Autodesk Inventor part; units mm, degrees
ref_plane "YZ Plane" through (0, 0, 0) normal (1, 0, 0) x (0, 1, 0)
ref_plane "XZ Plane" through (0, 0, 0) normal (0, 1, 0) x (-1, 0, 0)
ref_plane "XY Plane" through (0, 0, 0) normal (0, 0, 1) x (1, 0, 0)
sketch "Sketch1" plane through (0, 0, 0) normal (0, 0, 1) x (1, 0, 0)
  line L0 (0, 0) -> (27, 0) construction
  line L1 (27, 0) -> (27, 27)
  line L2 (27, 27) -> (0, 27)
  line L3 (0, 27) -> (0, 0) construction
  line L4 (-27, 0) -> (-27, 27)
  line L5 (-27, 27) -> (0, 27)
  line L6 (27, 0) -> (27, -27)
  line L7 (27, -27) -> (0, -27)
  line L8 (-27, -27) -> (0, -27)
  line L9 (-27, 0) -> (-27, -27)
  dimension "d0" = 27
extrude "Extrusion1" add sketch "Sketch1" along normal mid plane 138
sketch "Sketch2" plane through (0, 0, 69) normal (0, 0, 1) x (1, 0, 0)
  line L0 (27, -27) -> (27, 27)
  line L1 (27, 27) -> (-27, 27)
  line L2 (-27, 27) -> (-27, -27)
  line L3 (-27, -27) -> (27, -27)
  circle A0 centre (0, 0) radius 27
extrude "Extrusion2" cut sketch "Sketch2" against normal blind 30 contours L3 A0 L0 | A0 L1 L0 | L3 L2 A0 | A0 L2 L1
sketch "Sketch3" plane through (-27, -27, -69) normal (0, -1, 0) x (1, 0, 0)
  line L0 (54, 108) -> (54, 0)
  circle A0 centre (27, 69) radius 27
extrude "Extrusion3" add sketch "Sketch3" along normal blind 12
move or copy body "Move Body1" bodies to move or copy 1 copy no rotation origin (0, 0, 0) rotation axis (1, 0, 0) rotation angle 90
move or copy body "Move Body2" bodies to move or copy 1 copy no rotation origin (0, 0, 0) rotation axis (0, 0, 1) rotation angle 90
properties part number "Sholder_Roll"
CAD build for the part. Positions are in the model's coordinates, mm. A direction names the side the tool comes from. Give positions to 0.01 mm unless a question says otherwise; leave off trailing zeros. Order: outer loops, then holes, each group sorted by start corner. A loop starts at its lowest first (then second) coordinate and runs counter-clockwise, first axis right, second up. Notation, with made-up numbers: M 64,25.25 L 97,25.25 A36 ccw 97,63.25 Z; hole C -2,-14.5 d2. An arc over 180 degrees is marked long. Put each result on its own line as item: value. Start each with the question number.
(1) Saw through at C-C, the plane y = 9.5. Write the cut outline in (x, z), then the cut area to 3 significant figures.
(2) Flat gauge pins, fed straight in: pin 1 Ø2 at (y, z) = (19.5, -30) entering from +X; pin 2 Ø3 at (x, y) = (-43.5, -9) entering from -Z; pin 3 Ø8 at (x, y) = (54, 18.5) entering from +Z. Where does each tip first touch, or does it go through?
(3) Saw through at D-D, the plane x = -39. Write the cut outline in (y, z), then the cut area to 3 significant figures.
(4) Drill centre lines: line 1 along Z through (x, y) = (-25, 22.5); line 2 along X through (y, z) = (21, -20.5). Where is each one in solid material? Low to high.
(5) Saw through at B-B, the plane x = -16. Write the cut outline in (y, z), then the cut area to 3 significant figures.
(6) Saw through at A-A, the plane y = -3.5. Write the cut outline in (x, z), then the cut area to 3 significant figures.
(7) Which spindle directions (+Z, -Z, +X, -X, +Y, -Y) get a long thin tool onto all of the face, cutting with end or side? Do faces 1 (the flat face through (39, -22, -20)), 2 (the flat face through (39, 21, -21)), 3 (the flat face through (39, -22, 21)), 4 (the cylindrical face through (26.36, -5.85, -32.92)). Say none if no direction does.
Check result:
1. outline: M -69,-27 L -25.27,-27 L -25.27,-39 L 25.27,-39 L 25.27,-27 L 39,-27 L 39,-25.27 L 69,-25.27 L 69,25.27 L 39,25.27 L 39,27 L -69,27 Z
1. area: 7,950 mm2
2. pin 1: stops at x = 19.67
2. pin 2: stops at z = -27
2. pin 3: stops at z = 22.78
3. outline: M -27,-27 L 27,-27 L 27,27 L -27,27 Z
3. area: 2,920 mm2
4. line 1: z = -27 to 27
4. line 2: x = -69 to 39
5. outline: M -27,-27 L -21.75,-27 L -21.75,-39 L 21.75,-39 L 21.75,-27 L 27,-27 L 27,27 L -27,27 Z
5. area: 3,440 mm2
6. outline: M -69,-27 L -26.77,-27 L -26.77,-39 L 26.77,-39 L 26.77,-27 L 39,-27 L 39,-26.77 L 69,-26.77 L 69,26.77 L 39,26.77 L 39,27 L -69,27 Z
6. area: 8,080 mm2
7. face 1: -Z, +X, -Y
7. face 2: -Z, +X, +Y
7. face 3: +Z, +X, -Y
7. face 4: -Z
